```python
from build123d import *

# Parameters (mm, degrees)
SKETCH_1_W               = 5
SKETCH_1_H               = 19
EXTRUDE_1_DEPTH          = 32.5
EXTRUDE_1_DEPTH_BACK     = 32.5
SKETCH_2_R               = 10
CUT_EXTRUDE_1_DEPTH      = 19
SKETCH_3_R               = 1.5
CUT_EXTRUDE_2_DEPTH      = 6
SKETCH_4_R               = 1.5
CUT_EXTRUDE_3_DEPTH      = 66
CUT_EXTRUDE_4_DEPTH      = 1
CUT_EXTRUDE_4_DEPTH_BACK = 47.5
SKETCH_6_W               = 33
SKETCH_6_H               = 13.5
CUT_EXTRUDE_5_DEPTH      = 10
FILLET_3_R               = 5


with BuildPart() as part:
    # Эскиз1 → Бобышка-Вытянуть1 (new body, two sides)
    with BuildSketch(Plane.XY) as extrude_1_sk:
        Polygon((46.5, 41), (5, 41), (5, 0), (0, 0), (0, 46), (46.5, 46), align=None)
        with Locations((2.5, -9.5)):
            Rectangle(SKETCH_1_W, SKETCH_1_H)
    extrude(amount=EXTRUDE_1_DEPTH)
    extrude(extrude_1_sk.sketch, amount=-EXTRUDE_1_DEPTH_BACK)

    # Эскиз2 → Вырез-Вытянуть1 (cut)
    with BuildSketch(Plane(origin=(5, 0, 0), x_dir=(0, 0, -1), z_dir=(1, 0, 0))):
        Circle(SKETCH_2_R)
    extrude(amount=-CUT_EXTRUDE_1_DEPTH, mode=Mode.SUBTRACT)

    # Эскиз3 → Вырез-Вытянуть2 (cut, through all)
    with BuildSketch(Plane(origin=(5, 0, 0), x_dir=(0, 0, -1), z_dir=(1, 0, 0))):
        with Locations((0, 14)):
            Circle(SKETCH_3_R)
        with Locations((7.5, 12.990381057)):
            Circle(SKETCH_3_R)
        with Locations((12.124355653, -7)):
            Circle(SKETCH_3_R)
        with Locations((7.5, -12.990381057)):
            Circle(SKETCH_3_R)
        with Locations((-12.124355653, -7)):
            Circle(SKETCH_3_R)
        with Locations((-15, 0)):
            Circle(SKETCH_3_R)
    extrude(amount=-CUT_EXTRUDE_2_DEPTH, mode=Mode.SUBTRACT)

    # Эскиз4 → Вырез-Вытянуть3 (cut, through all)
    with BuildSketch(Plane(origin=(0, 46, 0), x_dir=(1, 0, 0), z_dir=(0, 1, 0))):
        with Locations((15, 15)):
            Circle(SKETCH_4_R)
        with Locations((15, 5)):
            Circle(SKETCH_4_R)
        with Locations((25, 5)):
            Circle(SKETCH_4_R)
        with Locations((25, 15)):
            Circle(SKETCH_4_R)
        with Locations((25, -15)):
            Circle(SKETCH_4_R)
        with Locations((25, -5)):
            Circle(SKETCH_4_R)
        with Locations((15, -5)):
            Circle(SKETCH_4_R)
        with Locations((15, -15)):
            Circle(SKETCH_4_R)
        with BuildLine():
            Line((38.5, 27.5), (38.5, 23.5))
            ThreePointArc((38.5, 23.5), (40, 22), (41.5, 23.5))
            Line((41.5, 23.5), (41.5, 27.5))
            ThreePointArc((41.5, 27.5), (40, 29), (38.5, 27.5))
        make_face()
        with BuildLine():
            Line((38.5, -23.511442769), (38.5, -27.516419302))
            ThreePointArc((38.5, -27.516419302), (40.008164842, -29.000022466), (41.5, -27.5))
            Line((41.5, -27.5), (41.5, -23.488557231))
            ThreePointArc((41.5, -23.488557231), (39.988557231, -22), (38.5, -23.511442769))
        make_face()
    extrude(amount=-CUT_EXTRUDE_3_DEPTH, mode=Mode.SUBTRACT)

    # Эскиз5 → Вырез-Вытянуть4 (cut, two sides)
    with BuildSketch(Plane.ZY) as cut_extrude_4_sk:
        with BuildLine():
            ThreePointArc((3e-08, -19), (-13.435028832, -13.435028853), (-19, 0))
            Line((-19, 0), (-19, 40))
            Line((-19, 40), (-32.5, 40))
            Line((-32.5, 40), (-32.5, -19))
            Line((-32.5, -19), (3e-08, -19))
        make_face()
        with BuildLine():
            Line((19, 40), (19, 0))
            ThreePointArc((19, 0), (13.435028853, -13.435028832), (3e-08, -19))
            Line((3e-08, -19), (32.5, -19))
            Line((32.5, -19), (32.5, 40))
            Line((32.5, 40), (19, 40))
        make_face()
        Polygon((32.5, -19), (3e-08, -19), (-32.5, -19), (-32.5, 40), (-39.097198646, 40), (-39.097198646, -21.281436411), (42.016942769, -21.281436411), (42.016942769, 40), (32.5, 40), align=None)
    extrude(amount=CUT_EXTRUDE_4_DEPTH, mode=Mode.SUBTRACT)
    extrude(cut_extrude_4_sk.sketch, amount=-CUT_EXTRUDE_4_DEPTH_BACK, mode=Mode.SUBTRACT)

    # Эскиз6 → Вырез-Вытянуть5 (cut)
    with BuildSketch(Plane(origin=(0, 46, 0), x_dir=(1, 0, 0), z_dir=(0, 1, 0))):
        with Locations((16.5, 25.75)):
            Rectangle(SKETCH_6_W, SKETCH_6_H)
        with Locations((16.5, -25.75)):
            Rectangle(SKETCH_6_W, SKETCH_6_H)
    extrude(amount=-CUT_EXTRUDE_5_DEPTH, mode=Mode.SUBTRACT)

    # Скругление3
    fillet_3_edges = [part.edges().sort_by_distance(p)[0] for p in [
        (46.5, 43.5, 32.5),
        (33, 43.5, 19),
        (33, 43.5, 32.5),
        (33, 43.5, -32.5),
        (33, 43.5, -19),
        (46.5, 43.5, -32.5),
    ]]
    fillet(fillet_3_edges, radius=FILLET_3_R)


solid = part.part
```
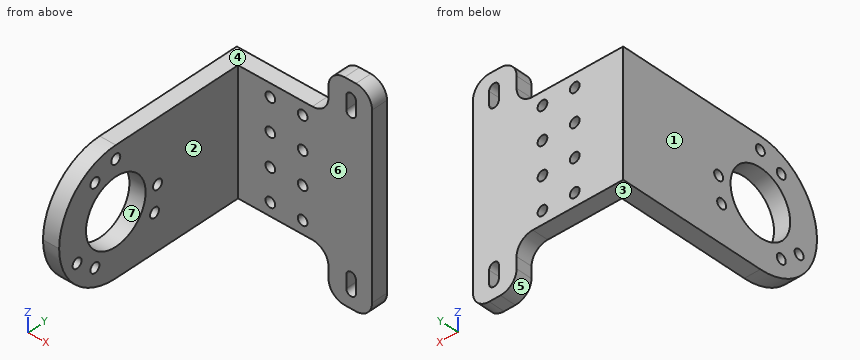
Build history of the part. All positions in model axes, mm. Face numbers are marked on the shaded views. A direction names the side the tool comes from. Give positions to 0.01 mm unless a question says otherwise; leave off trailing zeros. Loops run counter-clockwise (first coordinate to the right, second up) from the corner with the lowest first, then second, coordinate; pieces in that order, holes last. Notation, with made-up numbers: (36, 59) -> (82, 59) arc R29 cw to (82, 86) -> close; hole circle Ø1 at (-18, -2.5). An arc over 180 degrees is marked (long way). One line per question, with ' | ' between items.
Q1. Cut at A-A, the plane x = 25. Write the cut outline in (y, z), plus the area to 3 significant figures.
Filled sheet:
outline: (41, -19) -> (46, -19) -> (46, -16.5) -> (41, -16.5) -> close; (41, -13.5) -> (46, -13.5) -> (46, -6.5) -> (41, -6.5) -> close; (41, -3.5) -> (46, -3.5) -> (46, 3.5) -> (41, 3.5) -> close; (41, 6.5) -> (46, 6.5) -> (46, 13.5) -> (41, 13.5) -> close; (41, 16.5) -> (46, 16.5) -> (46, 19) -> (41, 19) -> close | area: 130 mm²
Q2. Cut at C-C, the plane y = -7. Write the cut outline in (x, z).
Filled sheet:
outline: (0, -17.66) -> (5, -17.66) -> (5, -13.62) -> (0, -13.62) -> close; (0, -10.62) -> (5, -10.62) -> (5, -7.14) -> (0, -7.14) -> close; (0, 7.14) -> (5, 7.14) -> (5, 10.62) -> (0, 10.62) -> close; (0, 13.62) -> (5, 13.62) -> (5, 17.66) -> (0, 17.66) -> close
Q3. Cut at D-D, the plane y = 9. Write the cut outline in (x, z).
Filled sheet:
outline: (0, -19) -> (5, -19) -> (5, -4.36) -> (0, -4.36) -> close; (0, 4.36) -> (5, 4.36) -> (5, 19) -> (0, 19) -> close
Q4. Cut at B-B, the plane z = 2.5. Write the cut outline in (x, y), plus the area to 3 significant figures.
Filled sheet:
outline: (0, -18.83) -> (5, -18.83) -> (5, -9.68) -> (0, -9.68) -> close; (0, 9.68) -> (5, 9.68) -> (5, 41) -> (46.5, 41) -> (46.5, 46) -> (0, 46) -> close | area: 435 mm²
Q5. Pull direction Z, two halves, no side cores. Call the marked faces 4, 5, 6 and 7: pulls with the +Z half, pulls with the -Z half, needs draft (parallel to the pull), parting line crosses it, or undercut.
Filled sheet:
face 4: pulls with the +Z half | face 5: pulls with the -Z half | face 6: needs draft | face 7: undercut
Q6. Drop flat-ended pins along their axis: pin 1 (2.5 mm diameter, centred on y = -7, z = -12.12, fed in from +X); pin 2 (6 mm diameter, centred on y = 18, z = -7, fed in from +X); pin 3 (1 mm diameter, centred on x = 32.5, z = 8, fed in from -Y); pin 4 (1.2 mm diameter, centred on y = 44.5, z = -24.5, fed in from -X). Give the stop position or say it passes through.
Filled sheet:
pin 1: passes through | pin 2: stops at x = 5 | pin 3: stops at y = 41 | pin 4: stops at x = 33
Q7. Tool access for the marked faces 1, 2 and 3: list every direction of +Z, -Z, +X, -X, +Y, -Y with a clear straight run to the whole face (end or side of a thin tool).
Filled sheet:
face 1: +Z, -Z, -X, +Y, -Y | face 2: +Z, -Z, +X, -Y | face 3: -Z, -X, +Y, -Y
Q8. Drill centre lines: line 1 along X through (y, z) = (42, 5); line 2 along Z through (x, y) = (15, 43.95); line 3 along X through (y, z) = (43.5, -6). Where is each one in solid material? Low to high. Write a range as [from, to].
Filled sheet:
line 1: x = [0, 13.5], [16.5, 23.5], [26.5, 46.5] | line 2: z = [-19, -16.5], [-13.5, -6.5], [-3.5, 3.5], [6.5, 13.5], [16.5, 19] | line 3: x = [0, 13.88], [16.12, 23.88], [26.12, 46.5]
